from build123d import *

# Parameters (mm, degrees)
F0_R     = 25.4
F0_R_2   = 23.495
F1_DEPTH = 6.35
F2_DEPTH = 2.54
F4_DEPTH = 2.54


with BuildPart() as f1:
    # F0 (on Top) → F1 (new body)
    with BuildSketch(Plane.XY):
        Circle(F0_R)
        Circle(F0_R_2, mode=Mode.SUBTRACT)
        Circle(F0_R_2)
        with BuildLine():
            ThreePointArc((19.4312153991, 10.7878864062), (21.5152200459, 5.5718875955), (22.225, 0))
            ThreePointArc((22.225, 0), (21.5152200459, -5.5718875955), (19.4312153991, -10.7878864062))
            ThreePointArc((19.4312153991, -10.7878864062), (14.5899693593, -16.7655426126), (8.001, -20.7348649381))
            ThreePointArc((8.001, -20.7348649381), (7.6843906394, -20.8542745139), (7.366, -20.9688499685))
            ThreePointArc((7.366, -20.9688499685), (5.7943813589, -21.4563689768), (4.191, -21.8262718759))
            ThreePointArc((4.191, -21.8262718759), (-1.3103135445, -22.1863404692), (-6.731, -21.1812243272))
            ThreePointArc((-6.731, -21.1812243272), (-7.3693802437, -20.9676622403), (-8.001, -20.7348649381))
            ThreePointArc((-8.001, -20.7348649381), (-14.9111451119, -16.480545393), (-19.833461849, -10.0291782357))
            ThreePointArc((-19.833461849, -10.0291782357), (-21.420808455, -5.9244907069), (-22.1682310695, -1.5875))
            ThreePointArc((-22.1682310695, -1.5875), (-18.7647973594, 11.9093662746), (-8.001, 20.7348649381))
            ThreePointArc((-8.001, 20.7348649381), (-7.3693802437, 20.9676622403), (-6.731, 21.1812243272))
            ThreePointArc((-6.731, 21.1812243272), (-1.3103135445, 22.1863404692), (4.191, 21.8262718759))
            ThreePointArc((4.191, 21.8262718759), (5.7943813589, 21.4563689768), (7.366, 20.9688499685))
            ThreePointArc((7.366, 20.9688499685), (7.6843906394, 20.8542745139), (8.001, 20.7348649381))
            ThreePointArc((8.001, 20.7348649381), (14.5899693593, 16.7655426126), (19.4312153991, 10.7878864062))
        make_face(mode=Mode.SUBTRACT)
        with BuildLine():
            Line((7.366, 17.5682823292), (4.191, 21.8262718759))
            ThreePointArc((4.191, 21.8262718759), (-1.3103135445, 22.1863404692), (-6.731, 21.1812243272))
            Line((-6.731, 21.1812243272), (-6.731, 14.3932823292))
            Line((-6.731, 14.3932823292), (-6.7315069765, 1.5621306643))
            Line((-6.7315069765, 1.5621306643), (-6.731, -1.5875))
            Line((-6.731, -1.5875), (-6.731, -21.1812243272))
            ThreePointArc((-6.731, -21.1812243272), (-1.3103135445, -22.1863404692), (4.191, -21.8262718759))
            Line((4.191, -21.8262718759), (7.366, -17.5682823292))
            Line((7.366, -17.5682823292), (7.366, -1.5875))
            Line((7.366, -1.5875), (7.366, 1.5875))
            Line((7.366, 1.5875), (7.366, 17.5682823292))
        make_face()
        with BuildLine():
            Line((-4.191, 1.5875), (-4.191, 18.5832725589))
            ThreePointArc((-4.191, 18.5832725589), (-0.3670330457, 19.0464638908), (3.4719400554, 18.7309405063))
            Line((3.4719400554, 18.7309405063), (4.191, 17.5682823292))
            Line((4.191, 17.5682823292), (4.191, -17.5672725589))
            Line((4.191, -17.5672725589), (3.3001679253, -18.7619666257))
            ThreePointArc((3.3001679253, -18.7619666257), (-0.4542888274, -19.0445824754), (-4.191, -18.5832725589))
            Line((-4.191, -18.5832725589), (-4.191, -1.5875))
            Line((-4.191, -1.5875), (-4.191, 1.5875))
        make_face(mode=Mode.SUBTRACT)
        with BuildLine():
            Line((-8.001, 14.3932823292), (-8.001, 20.7348649381))
            ThreePointArc((-8.001, 20.7348649381), (-18.7647973594, 11.9093662746), (-22.1682310695, -1.5875))
            Line((-22.1682310695, -1.5875), (-18.9837389297, -1.5875))
            Line((-18.9837389297, -1.5875), (-10.541, -1.5875))
            Line((-10.541, -1.5875), (-10.541, -15.8678864062))
            ThreePointArc((-10.541, -15.8678864062), (-13.6836612477, -13.2536755226), (-16.1962367208, -10.0291782357))
            Line((-16.1962367208, -10.0291782357), (-19.833461849, -10.0291782357))
            ThreePointArc((-19.833461849, -10.0291782357), (-14.9111451119, -16.480545393), (-8.001, -20.7348649381))
            Line((-8.001, -20.7348649381), (-8.001, -1.5875))
            Line((-8.001, -1.5875), (-8.001, 1.5875))
            Line((-8.001, 1.5875), (-18.9837389297, 1.5875))
            ThreePointArc((-18.9837389297, 1.5875), (-16.3984728311, 9.6949775042), (-10.541, 15.8678864062))
            Line((-10.541, 15.8678864062), (-10.541, 14.3932823292))
            Line((-10.541, 14.3932823292), (-8.001, 14.3932823292))
        make_face()
        with BuildLine():
            Line((15.7010829845, 10.7878864062), (19.4312153991, 10.7878864062))
            ThreePointArc((19.4312153991, 10.7878864062), (14.5899693593, 16.7655426126), (8.001, 20.7348649381))
            Line((8.001, 20.7348649381), (8.001, -20.7348649381))
            ThreePointArc((8.001, -20.7348649381), (14.5899693593, -16.7655426126), (19.4312153991, -10.7878864062))
            Line((19.4312153991, -10.7878864062), (15.7010829845, -10.7878864062))
            ThreePointArc((15.7010829845, -10.7878864062), (13.3646298056, -13.5753147351), (10.541, -15.8678864062))
            Line((10.541, -15.8678864062), (10.541, -1.5875))
            Line((10.541, -1.5875), (14.478, -1.5875))
            Line((14.478, -1.5875), (14.478, 1.5875))
            Line((14.478, 1.5875), (10.541, 1.5875))
            Line((10.541, 1.5875), (10.541, 15.8678864062))
            ThreePointArc((10.541, 15.8678864062), (13.3646298056, 13.5753147351), (15.7010829845, 10.7878864062))
        make_face()
        with BuildLine():
            Line((8.001, -20.7348649381), (8.001, 20.7348649381))
            ThreePointArc((8.001, 20.7348649381), (7.6843906394, 20.8542745139), (7.366, 20.9688499685))
            Line((7.366, 20.9688499685), (7.366, 17.5682823292))
            Line((7.366, 17.5682823292), (7.366, 1.5875))
            Line((7.366, 1.5875), (7.366, -1.5875))
            Line((7.366, -1.5875), (7.366, -17.5682823292))
            Line((7.366, -17.5682823292), (7.366, -20.9688499685))
            ThreePointArc((7.366, -20.9688499685), (7.6843906394, -20.8542745139), (8.001, -20.7348649381))
        make_face()
        with BuildLine():
            ThreePointArc((-8.001, -20.7348649381), (-7.3693802437, -20.9676622403), (-6.731, -21.1812243272))
            Line((-6.731, -21.1812243272), (-6.731, -1.5875))
            Line((-6.731, -1.5875), (-7.366, -1.5875))
            Line((-7.366, -1.5875), (-8.001, -1.5875))
            Line((-8.001, -1.5875), (-8.001, -20.7348649381))
        make_face()
        with BuildLine():
            Line((-6.731, 14.3932823292), (-6.731, 21.1812243272))
            ThreePointArc((-6.731, 21.1812243272), (-7.3693802437, 20.9676622403), (-8.001, 20.7348649381))
            Line((-8.001, 20.7348649381), (-8.001, 14.3932823292))
            Line((-8.001, 14.3932823292), (-7.366, 14.3932823292))
            Line((-7.366, 14.3932823292), (-6.731, 14.3932823292))
        make_face()
        Polygon((-6.7315069765, 1.5621306643), (-6.731, 14.3932823292), (-7.366, 14.3932823292), (-7.366, 1.5875), align=None)
        Polygon((-7.366, -1.5875), (-6.731, -1.5875), (-6.7315069765, 1.5621306643), (-7.366, 1.5875), (-8.001, 1.5875), (-8.001, -1.5875), align=None)
    extrude(amount=-F1_DEPTH)

    # F0 (on Top) → F2 (cut)
    with BuildSketch(Plane.XY):
        Circle(F0_R_2)
        with BuildLine():
            ThreePointArc((19.4312153991, 10.7878864062), (21.5152200459, 5.5718875955), (22.225, 0))
            ThreePointArc((22.225, 0), (21.5152200459, -5.5718875955), (19.4312153991, -10.7878864062))
            ThreePointArc((19.4312153991, -10.7878864062), (14.5899693593, -16.7655426126), (8.001, -20.7348649381))
            ThreePointArc((8.001, -20.7348649381), (7.6843906394, -20.8542745139), (7.366, -20.9688499685))
            ThreePointArc((7.366, -20.9688499685), (5.7943813589, -21.4563689768), (4.191, -21.8262718759))
            ThreePointArc((4.191, -21.8262718759), (-1.3103135445, -22.1863404692), (-6.731, -21.1812243272))
            ThreePointArc((-6.731, -21.1812243272), (-7.3693802437, -20.9676622403), (-8.001, -20.7348649381))
            ThreePointArc((-8.001, -20.7348649381), (-14.9111451119, -16.480545393), (-19.833461849, -10.0291782357))
            ThreePointArc((-19.833461849, -10.0291782357), (-21.420808455, -5.9244907069), (-22.1682310695, -1.5875))
            ThreePointArc((-22.1682310695, -1.5875), (-18.7647973594, 11.9093662746), (-8.001, 20.7348649381))
            ThreePointArc((-8.001, 20.7348649381), (-7.3693802437, 20.9676622403), (-6.731, 21.1812243272))
            ThreePointArc((-6.731, 21.1812243272), (-1.3103135445, 22.1863404692), (4.191, 21.8262718759))
            ThreePointArc((4.191, 21.8262718759), (5.7943813589, 21.4563689768), (7.366, 20.9688499685))
            ThreePointArc((7.366, 20.9688499685), (7.6843906394, 20.8542745139), (8.001, 20.7348649381))
            ThreePointArc((8.001, 20.7348649381), (14.5899693593, 16.7655426126), (19.4312153991, 10.7878864062))
        make_face(mode=Mode.SUBTRACT)
        with BuildLine():
            Line((-6.731, 14.3932823292), (-6.731, 21.1812243272))
            ThreePointArc((-6.731, 21.1812243272), (-7.3693802437, 20.9676622403), (-8.001, 20.7348649381))
            Line((-8.001, 20.7348649381), (-8.001, 14.3932823292))
            Line((-8.001, 14.3932823292), (-7.366, 14.3932823292))
            Line((-7.366, 14.3932823292), (-6.731, 14.3932823292))
        make_face()
        Polygon((-6.7315069765, 1.5621306643), (-6.731, 14.3932823292), (-7.366, 14.3932823292), (-7.366, 1.5875), align=None)
        Polygon((-7.366, -1.5875), (-6.731, -1.5875), (-6.7315069765, 1.5621306643), (-7.366, 1.5875), (-8.001, 1.5875), (-8.001, -1.5875), align=None)
        with BuildLine():
            ThreePointArc((-8.001, -20.7348649381), (-7.3693802437, -20.9676622403), (-6.731, -21.1812243272))
            Line((-6.731, -21.1812243272), (-6.731, -1.5875))
            Line((-6.731, -1.5875), (-7.366, -1.5875))
            Line((-7.366, -1.5875), (-8.001, -1.5875))
            Line((-8.001, -1.5875), (-8.001, -20.7348649381))
        make_face()
        with BuildLine():
            Line((8.001, -20.7348649381), (8.001, 20.7348649381))
            ThreePointArc((8.001, 20.7348649381), (7.6843906394, 20.8542745139), (7.366, 20.9688499685))
            Line((7.366, 20.9688499685), (7.366, 17.5682823292))
            Line((7.366, 17.5682823292), (7.366, 1.5875))
            Line((7.366, 1.5875), (7.366, -1.5875))
            Line((7.366, -1.5875), (7.366, -17.5682823292))
            Line((7.366, -17.5682823292), (7.366, -20.9688499685))
            ThreePointArc((7.366, -20.9688499685), (7.6843906394, -20.8542745139), (8.001, -20.7348649381))
        make_face()
    extrude(amount=-F2_DEPTH, mode=Mode.SUBTRACT)

    # F3 (on face) → F4 (join)
    with BuildSketch(Plane(origin=(0, 0, -6.35), x_dir=(1, 0, 0), z_dir=(0, 0, -1))):
        with BuildLine():
            ThreePointArc((-4.4279512894, -25.0110625), (-5.3678907079, -24.826311634), (-6.3001953095, -24.60625))
            ThreePointArc((-6.3001953095, -24.60625), (0, -31.75), (6.3001953095, -24.60625))
            ThreePointArc((6.3001953095, -24.60625), (5.3678907079, -24.826311634), (4.4279512894, -25.0110625))
            ThreePointArc((4.4279512894, -25.0110625), (0, -29.845), (-4.4279512894, -25.0110625))
        make_face()
    extrude(amount=-F4_DEPTH)


solid = f1.part
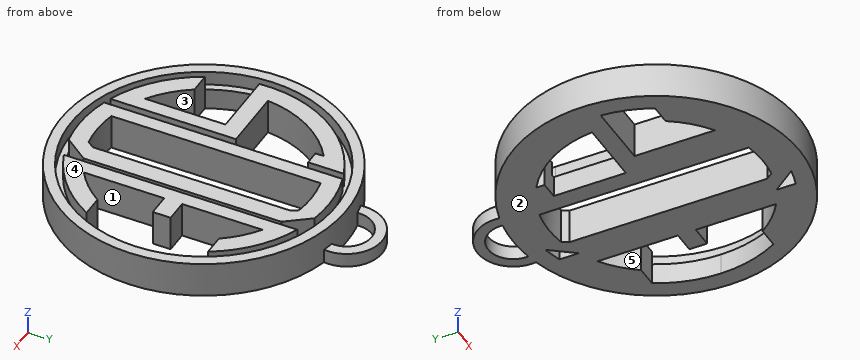
Read the model definition and answer for the solid it produces. Units are mm, in the model's axes. Face numbers are marked on the shaded views. A direction names the side the tool comes from. Round coordinates to 2 decimals unless told otherwise and drop trailing zeros. Write each loop counter-clockwise with the first axis right and the second up, starting at its lowest first coordinate (ties: lowest second). Pieces come first, ordered by that corner, then holes. Notation, with made-up numbers: M 54,56 L 87,56 A11 ccw 87,71 Z; hole C -19.75,58.5 d9. An arc over 180 degrees is marked long. Use a Markdown table: item, result.
1) For a pull along Y with two mould halves and no side action, classify the marked faces 3, 4 and 5 as pulls with the +Y half, pulls with the -Y half, needs draft (parallel to the pull), parting line crosses it, or undercut.
Answers follow:
| item | result |
|---|---|
| face 3 | undercut |
| face 4 | needs draft |
| face 5 | undercut |
2) The part is cut by section C-C (x = 13). Write down the section's boundary in (y, z), plus the area to 3 significant figures.
Answers follow:
| item | result |
|---|---|
| outline | M -21.82,-6.35 L -13.92,-6.35 L -13.92,0 L -18.03,0 L -18.03,-2.54 L -19.57,-2.54 L -19.57,0 L -21.82,0 Z; M -1.59,-6.35 L 1.59,-6.35 L 1.59,0 L -1.59,0 Z; M 13.92,-6.35 L 21.82,-6.35 L 21.82,0 L 19.57,0 L 19.57,-2.54 L 18.03,-2.54 L 18.03,0 L 13.92,0 Z |
| area | 113 mm2 |
3) Straight lines are drawn through the part: line 1 along Y through (x, z) = (0, -1) (3 decimals); line 2 along X through (y, z) = (4, -4.25); line 3 along X through (y, z) = (10.5, -2). For each, find the intervals that lie inside material, in ascending order. Write a range as [from, to].
Answers follow:
| item | result |
|---|---|
| line 1 | y = [-25.4, -23.495], [-22.225, -19.05], [19.05, 22.225], [23.495, 25.4] |
| line 2 | x = [-25.08, -18.63], [-7.37, -4.19], [4.19, 10.54], [21.86, 25.08] |
| line 3 | x = [-23.13, -21.02], [-19.59, -15.9], [-6.73, -4.19], [4.19, 7.37], [8, 10.54], [21.02, 23.13] |
4) Flat-ended cylindrical pins translate along their axes: pin 1 (2 mm diameter, centred on y = -2, z = -2, fed in from +X); pin 2 (8 mm diameter, centred on x = -1, y = -5, fed in from +Z); pin 3 (3 mm diameter, centred on x = 17.5, z = -3.5, fed in from -Y); pin 4 (3 mm diameter, centred on x = -12.5, z = -2.5, fed in from +Y). Find the tip coordinate at first contact, or state that the pin passes through.
Answers follow:
| item | result |
|---|---|
| pin 1 | stops at x = 25.38 |
| pin 2 | stops at z = 0 |
| pin 3 | stops at y = -19.73 |
| pin 4 | stops at y = 22.89 |
5) A tool of negligible diameter and unlimited length cuts with its end or side. For the marked faces 1 and 2, from which of +Z, -Z, +X, -X, +Y, -Y can it reach the whole face along a straight path? Write none if from no direction.
Answers follow:
| item | result |
|---|---|
| face 1 | +Z, -Z |
| face 2 | -Z, +X, -X, +Y, -Y |
6) The part is cut by section B-B (y = -14.5). Give the number of separate pieces and of enclosed holes in the cut face, plus the area to 3 significant figures.
Answers follow:
| item | result |
|---|---|
| separate pieces | 4 |
| enclosed holes | 0 |
| area | 175 mm2 |
7) The part is cut by section A-A (x = 0). Write down the section's boundary in (y, z) (3 decimals).
Answers follow:
| item | result |
|---|---|
| outline | M -25.4,-6.35 L -19.05,-6.35 L -19.05,0 L -22.225,0 L -22.225,-2.54 L -23.495,-2.54 L -23.495,0 L -25.4,0 Z; M 19.05,-6.35 L 25.4,-6.35 L 25.4,0 L 23.495,0 L 23.495,-2.54 L 22.225,-2.54 L 22.225,0 L 19.05,0 Z; M 29.845,-6.35 L 31.75,-6.35 L 31.75,-3.81 L 29.845,-3.81 Z |
